Here's the drawing with two shaded views (mm, measured from the low corner). I have some questions. A direction names the side the tool comes from. Round coordinates to 2 decimals unless told otherwise and drop trailing zeros. Loops run counter-clockwise (first coordinate to the right, second up) from the corner with the lowest first, then second, coordinate; pieces in that order, holes last.
(1) Which directions (+Z, -Z, +X, -X, +Y, -Y) give clear straight access to the entire face, cutting with the end or side of a thin tool? Please do the marked faces 5 and 6.
(2) Will these pins go through, and if not, where does the flat tip stop? pin 1 Ø10 at (x, z) = (7, 4.5) entering from +Y; pin 2 Ø1.8 at (y, z) = (10.34, 2.04) entering from -X; pin 3 Ø5 at (x, z) = (8, 15.5) entering from +Y; pin 4 Ø0.8 at (x, z) = (1, 26.5) entering from -Y.
(3) I want a section at D-D on x = 6. Write out the boundary of the cut face in (y, z).
(4) Thinking about a two-plate mould opening in X: for the marked faces 1, 2, 3 and 4, which applies, released by +X, released by -X, zero draft, split by the parting line, or undercut?
(5) I want a section at A-A on z = 27. Write out the boundary of the cut face in (x, y).
(6) If I drill on line 1 along X through (y, z) = (7.25, 11.5); line 2 along X through (y, z) = (1.2, 22.5) (1 decimal); line 3 along Z through (x, y) = (1.15, 10.34), over which ranges is the centre line in solid material (lowest first)?
(7) I want a section at B-B on z = 22.5. Write out the boundary of the cut face in (x, y).
(8) I want a section at C-C on y = 5.5. Write out the boundary of the cut face in (x, z).
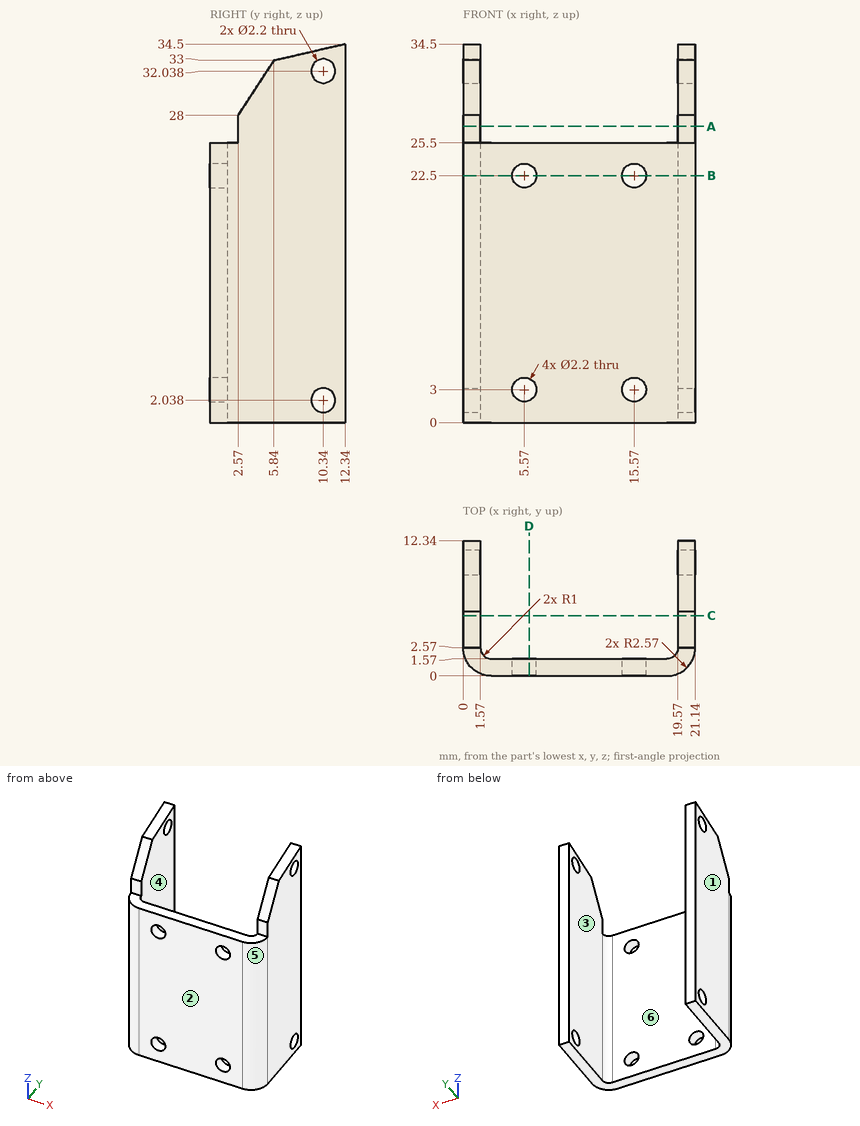
Filled sheet:
1. face 5: +Z, -Z, +X, -Y
1. face 6: +Z, -Z, +Y
2. pin 1: stops at y = 1.75
2. pin 2: passes through
2. pin 3: stops at y = 1.57
2. pin 4: stops at y = 2.57
3. outline: (0, 0) - (1.57, 0) - (1.57, 1.99) - (0, 1.99) - close; (0, 4.01) - (1.57, 4.01) - (1.57, 21.49) - (0, 21.49) - close; (0, 23.51) - (1.57, 23.51) - (1.57, 25.5) - (0, 25.5) - close
4. face 1: released by -X
4. face 2: zero draft
4. face 3: undercut
4. face 4: undercut
5. outline: (0, 2.57) - (1.57, 2.57) - (1.57, 12.34) - (0, 12.34) - close; (19.57, 2.57) - (21.14, 2.57) - (21.14, 12.34) - (19.57, 12.34) - close
6. line 1: x = 0 to 1.57, 19.57 to 21.14
6. line 2: x = 0.4 to 4.5, 6.7 to 14.5, 16.7 to 20.7
6. line 3: z = 0 to 0.94, 3.14 to 30.94, 33.14 to 34.04
7. outline: (0, 2.57) arc R2.57 ccw to (2.57, 0) - (4.47, 0) - (4.47, 1.57) - (2.57, 1.57) arc R1 cw to (1.57, 2.57) - (1.57, 12.34) - (0, 12.34) - close; (6.67, 0) - (14.47, 0) - (14.47, 1.57) - (6.67, 1.57) - close; (16.67, 0) - (18.57, 0) arc R2.57 ccw to (21.14, 2.57) - (21.14, 12.34) - (19.57, 12.34) - (19.57, 2.57) arc R1 cw to (18.57, 1.57) - (16.67, 1.57) - close
8. outline: (0, 0) - (1.57, 0) - (1.57, 32.48) - (0, 32.48) - close; (19.57, 0) - (21.14, 0) - (21.14, 32.48) - (19.57, 32.48) - close
